from build123d import *

# Parameters (mm, degrees)
F2_R            = 5.5
F3_DEPTH        = 20.001
F3_COPIES_COUNT = 3
F4_R            = 2.5
F5_DEPTH        = 15
F5_COPIES_COUNT = 6


# Not quite as in the source:
# - a pattern or mirror of a feature is missing from the dataset's text; its kind, count and spacing are read off the source's solid


with BuildPart() as f1:
    # F0 (on Front) → F1 (revolve)
    with BuildSketch(Plane.XZ):
        Polygon((0, 70), (0, 29.148), (9.798351825, 26.5), (20, 26.5), (20, 70), align=None)
    revolve(axis=Axis((21.5308236951, 0, 0), (1, 0, 0)))

    # F2 (on face) → F3 (cut, through all)
    with BuildSketch(Plane(origin=(0, 0, 0), x_dir=(0, -1, 0), z_dir=(-1, 0, 0))):
        with Locations((30, 51.9615242271)):
            Circle(F2_R)
    f3 = extrude(amount=-F3_DEPTH, mode=Mode.SUBTRACT)

    # F3_copies: F3 ×3 about axis
    f3_copies_axis = Axis((0, 0, 0), (1, 0, 0))
    for i in range(1, F3_COPIES_COUNT):
        add(f3.rotate(f3_copies_axis, i * 360 / F3_COPIES_COUNT), mode=Mode.SUBTRACT)

    # F4 (on face) → F5 (cut)
    with BuildSketch(Plane.YZ.offset(20)):
        with Locations((-30.3108891325, 17.5)):
            Circle(F4_R)
    f5 = extrude(amount=-F5_DEPTH, mode=Mode.SUBTRACT)

    # F5_copies: F5 ×6 about axis
    f5_copies_axis = Axis((0, 0, 0), (1, 0, 0))
    for i in range(1, F5_COPIES_COUNT):
        add(f5.rotate(f5_copies_axis, i * 360 / F5_COPIES_COUNT), mode=Mode.SUBTRACT)


solid = f1.part
CAD build for the part. Positions are in the model's coordinates, mm. A direction names the side the tool comes from. Round coordinates to 2 decimals unless told otherwise and drop trailing zeros. Loops run counter-clockwise (first coordinate to the right, second up) from the corner with the lowest first, then second, coordinate; pieces in that order, holes last.
(1) Two-plate mould, pull along Y, no slides. Class faces 3 (the cylindrical face through (12.6, -1.15, 37.22)), 4 (the cylindrical face through (9.86, 42.594, -55.55)), 5 (the flat face through (20, -1, -30)): +Y half, -Y half, draft (parallel to the pull), parting line (faces both ways), or undercut.
(2) Wall check: line 1 along Y through (x, z) = (18.25, 16); line 2 along Z through (x, y) = (13.5, -30); line 3 along Z through (x, y) = (7, -25). Give the ranges that are in metal, low to high.
(3) Cut at C-C (x = 18). State how many separate pieces and enclosed holes the cut face has, plus the area to 3 significant figures.
(4) Cut at B-B (y = 60). Give the cut face in (x, z).
(5) Cut at A-A (z = 0). Give the cut face in (x, y).
(6) Drop flat-ended pins along their axis: pin 1 (12 mm diameter, centred on x = 9.5, y = -20, fed in from -Z); pin 2 (10 mm diameter, centred on x = 3, y = 46, fed in from +Z); pin 3 (4 mm diameter, centred on x = 13, z = -7.5, fed in from +Y). Give the stop position or say it passes through.
(7) Cut at D-D (z = 35). Give the cut face in (x, y), plus the area to 3 significant figures.
(8) Which spindle directions (+Z, -Z, +X, -X, +Y, -Y) get a long thin tool onto all of the face, cutting with end or side? Do faces 1 (the cylindrical face through (9.86, -35.246, -50.309)), 2 (the cylindrical face through (12.6, -31.5, -15.3)). Say none if no direction does.
Findings below:
1. face 3: undercut
1. face 4: parting line
1. face 5: draft
2. line 1: y = -68.15 to -32.31, -28.31 to -21.12, 21.12 to 28.31, 32.31 to 68.15
2. line 2: z = -63.25 to -57.46, -46.46 to -19.98, -15.02 to 15.02, 19.98 to 46.46, 57.46 to 63.25
2. line 3: z = -65.38 to -54.25, -49.67 to -10.86, 10.86 to 49.67, 54.25 to 65.38
3. separate pieces: 1
3. enclosed holes: 10
3. area: 12,800 mm2
4. outline: (0, -36.06) - (20, -36.06) - (20, -5.5) - (0, -5.5) - close; (0, 5.5) - (20, 5.5) - (20, 36.06) - (0, 36.06) - close
5. outline: (0, -70) - (20, -70) - (20, -26.5) - (9.8, -26.5) - (0, -29.15) - close; (0, 29.15) - (9.8, 26.5) - (20, 26.5) - (20, 54.5) - (0, 54.5) - close; (0, 65.5) - (20, 65.5) - (20, 70) - (0, 70) - close
6. pin 1: stops at z = -68.59
6. pin 2: stops at z = 56.74
6. pin 3: stops at y = 69.78
7. outline: (0, -60.62) - (20, -60.62) - (20, -2.5) - (5, -2.5) - (5, 2.5) - (20, 2.5) - (20, 60.62) - (0, 60.62) - close
7. area: 2,350 mm2
8. face 1: +X, -X
8. face 2: +X
